Autodesk Inventor part; units mm, degrees
ref_plane "YZ Plane" through (0, 0, 0) normal (1, 0, 0) x (0, 1, 0)
ref_plane "XZ Plane" through (0, 0, 0) normal (0, 1, 0) x (-1, 0, 0)
ref_plane "XY Plane" through (0, 0, 0) normal (0, 0, 1) x (1, 0, 0)
sketch "Sketch1" plane through (0, 0, 0) normal (0, 0, 1) x (1, 0, 0)
  line L0 (0, 4) -> (0, 26)
  line L1 (0, 26) -> (10, 26)
  line L2 (10, 26) -> (10, 30)
  line L3 (10, 30) -> (20, 30)
  line L4 (20, 30) -> (20, 26)
  line L5 (20, 26) -> (30, 26)
  line L6 (30, 26) -> (30, 4)
  line L7 (30, 4) -> (20, 4)
  line L8 (20, 4) -> (20, 0)
  line L9 (20, 0) -> (10, 0)
  line L10 (10, 0) -> (10, 4)
  line L11 (10, 4) -> (0, 4)
  point P0 (0, 0)
  dimension "d0" = 22
  dimension "d1" = 10
  dimension "d2" = 4
  dimension "d3" = 10
  dimension "d4" = 10
extrude "Extrusion1" add sketch "Sketch1" along normal blind 4
properties part number "innanverdurstubbur"
Source: CAD feature listing. Evaluate the final solid. Frame: model axes, mm. A direction names the side the tool comes from. Coordinates: 2 decimals unless noted, no trailing zeros. Loops run counter-clockwise (first coordinate to the right, second up) from the corner with the lowest first, then second, coordinate; pieces in that order, holes last. Notation, with made-up numbers: (4.25, 10.25) -> (51.25, 10.25) arc R28 ccw to (51.25, 30.25) -> close; hole circle Ø7 at (36, -18.75). An arc over 180 degrees is marked (long way). One line per item, written item: value. Start each with the question number.
Q1. Section query A-A, the plane z = 0.45. Return the cut outline in (x, y), and give its area (3 significant figures).
Q2. Line query: line 1 along Y through (x, z) = (9.5, 0.75); line 2 along X through (y, z) = (28.5, 0.5). Output: solid intervals per line, ascending.
Q3. Set-up query: faces 1 (the face through (10, 28, 2)), 2 (the face through (10, 2, 2)), 3 (the face through (20, 28, 2)), 4 (the face through (20, 2, 2)). Return all of +Z, -Z, +X, -X, +Y, -Y with unobstructed straight access to the full face (end or side cutting, diameter ignored); none if empty.
Q4. Section query B-B, the plane x = 6.75. Return the cut outline in (y, z), and give its area (3 significant figures).
Q5. Section query C-C, the plane y = 28.25. Return the cut outline in (x, z).
Q6. Contact query for flat-ended pins moving along their axis: P1, Ø2, axis at y = 2.5, z = 2.5, coming from the -X side; P2, Ø1.2, axis at x = 26.5, z = 1.5, coming from the +Y side. Output: stop coordinate, or through.
Results:
1. outline: (0, 4) -> (10, 4) -> (10, 0) -> (20, 0) -> (20, 4) -> (30, 4) -> (30, 26) -> (20, 26) -> (20, 30) -> (10, 30) -> (10, 26) -> (0, 26) -> close
1. area: 740 mm^2
2. line 1: 4 to 26
2. line 2: 10 to 20
3. face 1: +Z, -Z, -X, +Y
3. face 2: +Z, -Z, -X, -Y
3. face 3: +Z, -Z, +X, +Y
3. face 4: +Z, -Z, +X, -Y
4. outline: (4, 0) -> (26, 0) -> (26, 4) -> (4, 4) -> close
4. area: 88.0 mm^2
5. outline: (10, 0) -> (20, 0) -> (20, 4) -> (10, 4) -> close
6. P1: x = 10
6. P2: y = 26
